Here's how the part is built. I have some questions about the finished solid (model axes, mm). A direction names the side the tool comes from. Coordinates: 2 decimals unless noted, no trailing zeros. Loops run counter-clockwise (first coordinate to the right, second up) from the corner with the lowest first, then second, coordinate; pieces in that order, holes last. Notation, with made-up numbers: M -37.75,27.5 L -21.75,27.5 A37 cw -21.75,66.5 Z; hole C 53.25,31.5 d9. An arc over 180 degrees is marked long. Use CSV: the item, a comma, the result in double quotes. Start each with the question number.
Q1. Which directions (+Z, -Z, +X, -X, +Y, -Y) give clear straight access to the entire face, cutting with the end or side of a thin tool? Please do faces 1 (the cylindrical face through (0.66, 2.479, 47.485)), 2 (the conical face through (0.555, 187.98, 64.514)), 3 (the flat face through (0, 176, 60)), 4 (the flat face through (-17, 0, 32)), 5 (the flat face through (-7.5, 162, 32)).
Q2. If we section it at C-C (y = 125.5): Please give me the cut outline in (x, z).
Q3. If we mould it in two halves opening along Y, with no side actions, what happens to faces 6 (the cylindrical face through (0.76, 197.49, 32.18)), 7 (the flat face through (0, 95, 65)), 8 (the flat face through (7.5, 162, 32)), 9 (the flat face through (0, 5, 33))? For each: +Y half, -Y half, draft (parallel to the pull), parting line (faces both ways), or undercut.
Q4. If we section it at A-A (z = 12.5): Please give me the cut outline in (x, y), and give its area (3 significant figures).
Q5. Please list where these lines run through material, in increasing order: probe 1 along Y at (x, z) = (-3.25, 62.25); probe 2 along X at (y, z) = (145.75, 59); probe 3 along Y at (x, z) = (-3.25, 60.75). Write a range as [from, to].
Q6. For pin 1 Ø2.5 at (x, z) = (8, 33) entering from -Y; pin 2 Ø3 at (x, y) = (2, 178) entering from -Z; pin 3 Ø3 at (y, z) = (57.5, 23.5) entering from +X, each with a flat end and sliding along its axis, tell me the tip position at first contact or that it passes through.
Q7. If we section it at B-B (y = 78.5): Please give me the cut outline in (x, z).
from build123d import *

# Parameters (mm, degrees)
BOSS_EXTRUDE1_DEPTH = 65
CHAMFER1_SIZE       = 10
SKETCH2_R           = 15
CUT_EXTRUDE1_DEPTH  = 5
SKETCH3_R           = 1.5
CUT_EXTRUDE2_DEPTH  = 7.5
FILLET1_R           = 1
SKETCH4_W           = 15
SKETCH4_H           = 40
CUT_EXTRUDE3_DEPTH  = 55
SKETCH5_W           = 15
SKETCH5_H           = 27
SKETCH5_R           = 1.5
CUT_EXTRUDE4_DEPTH  = 209.416650007


with BuildPart() as part:
    # Sketch1 → Boss-Extrude1 (new body)
    with BuildSketch(Plane.XY):
        with BuildLine():
            Line((-37.5, 0), (37.5, 0))
            Line((37.5, 0), (34.995872386, 163.037509012))
            ThreePointArc((34.995872386, 163.037509012), (0, 197.5), (-34.995872386, 163.037509012))
            Line((-34.995872386, 163.037509012), (-37.5, 0))
        make_face()
    extrude(amount=BOSS_EXTRUDE1_DEPTH)

    # Chamfer1
    chamfer1_edges = [part.edges().sort_by_distance(p)[0] for p in [
        (-36.247936193, 81.518754506, 65),
        (36.247936193, 81.518754506, 65),
        (-36.247936193, 81.518754506, 0),
        (0, 197.5, 0),
        (36.247936193, 81.518754506, 0),
        (0, 197.5, 65),
    ]]
    chamfer(chamfer1_edges, length=CHAMFER1_SIZE)

    # Sketch2 → Cut-Extrude1 (cut)
    with BuildSketch(Plane(origin=(0, 0, 0), x_dir=(-1, 0, 0), z_dir=(0, -1, 0))):
        with Locations(Location((0, -32.5, 0), (0, 0, 90))):
            Circle(SKETCH2_R)
    extrude(amount=-CUT_EXTRUDE1_DEPTH, mode=Mode.SUBTRACT)

    # Sketch3 → Cut-Extrude2 (cut)
    with BuildSketch(Plane(origin=(0, 5, 0), x_dir=(-1, 0, 0), z_dir=(0, -1, 0))):
        with Locations(Location((0, -40, 0), (0, 0, 90))):
            Circle(SKETCH3_R)
        with Locations(Location((-7.5, -32.5, 0), (0, 0, 90))):
            Circle(SKETCH3_R)
        with Locations(Location((0, -25, 0), (0, 0, 90))):
            Circle(SKETCH3_R)
        with Locations(Location((7.5, -32.5, 0), (0, 0, 90))):
            Circle(SKETCH3_R)
    extrude(amount=-CUT_EXTRUDE2_DEPTH, mode=Mode.SUBTRACT)

    # Fillet1
    fillet1_edges = [part.edges().sort_by_distance(p)[0] for p in [
        (0, 5, 47.5),
        (0, 0, 47.5),
    ]]
    fillet(fillet1_edges, radius=FILLET1_R)

    # Sketch4 → Cut-Extrude3 (cut)
    with BuildSketch(Plane(origin=(0, 0, 0), x_dir=(-1, 0, 0), z_dir=(0, 0, -1))):
        with Locations((0, 162.5)):
            Rectangle(SKETCH4_W, SKETCH4_H)
    extrude(amount=-CUT_EXTRUDE3_DEPTH, mode=Mode.SUBTRACT)

    # Sketch5 → Cut-Extrude4 (cut, through all)
    with BuildSketch(Plane(origin=(0, 0, 55), x_dir=(-1, 0, 0), z_dir=(0, 0, -1))):
        with Locations((0, 162.5)):
            Rectangle(SKETCH5_W, SKETCH5_H)
        with Locations((-3.25, 179.25)):
            Circle(SKETCH5_R)
        with Locations((3.25, 179.25)):
            Circle(SKETCH5_R)
        with Locations((-3.25, 145.75)):
            Circle(SKETCH5_R)
        with Locations((3.25, 145.75)):
            Circle(SKETCH5_R)
    extrude(amount=-CUT_EXTRUDE4_DEPTH, mode=Mode.SUBTRACT)


solid = part.part
Results below:
1,face 1,"-Y"
1,face 2,"+Z, +Y"
1,face 3,"+Z, -Z"
1,face 4,"+Z, -Z, +X, -X, -Y"
1,face 5,"-Z"
2,outline,"M -35.57,10 L -25.57,0 L 25.57,0 L 35.57,10 L 35.57,55 L 25.57,65 L -25.57,65 L -35.57,55 Z"
3,face 6,"+Y half"
3,face 7,"draft"
3,face 8,"undercut"
3,face 9,"-Y half"
4,outline,"M -37.5,0 L 37.5,0 L 35,163.04 A35 ccw -35,163.04 Z; hole M -7.5,142.5 L 7.5,142.5 L 7.5,182.5 L -7.5,182.5 Z"
4,area,"13,100 mm^2"
5,probe 1,"[0, 144.25], [147.25, 149], [176, 177.75], [180.75, 190.06]"
5,probe 2,"[-31.26, -4.75], [-1.75, 1.75], [4.75, 31.26]"
5,probe 3,"[0, 144.25], [147.25, 149], [176, 177.75], [180.75, 191.57]"
6,pin 1,"y = 5"
6,pin 2,"z = 55"
6,pin 3,"x = 36.64"
7,outline,"M -36.29,10 L -26.29,0 L 26.29,0 L 36.29,10 L 36.29,55 L 26.29,65 L -26.29,65 L -36.29,55 Z"
